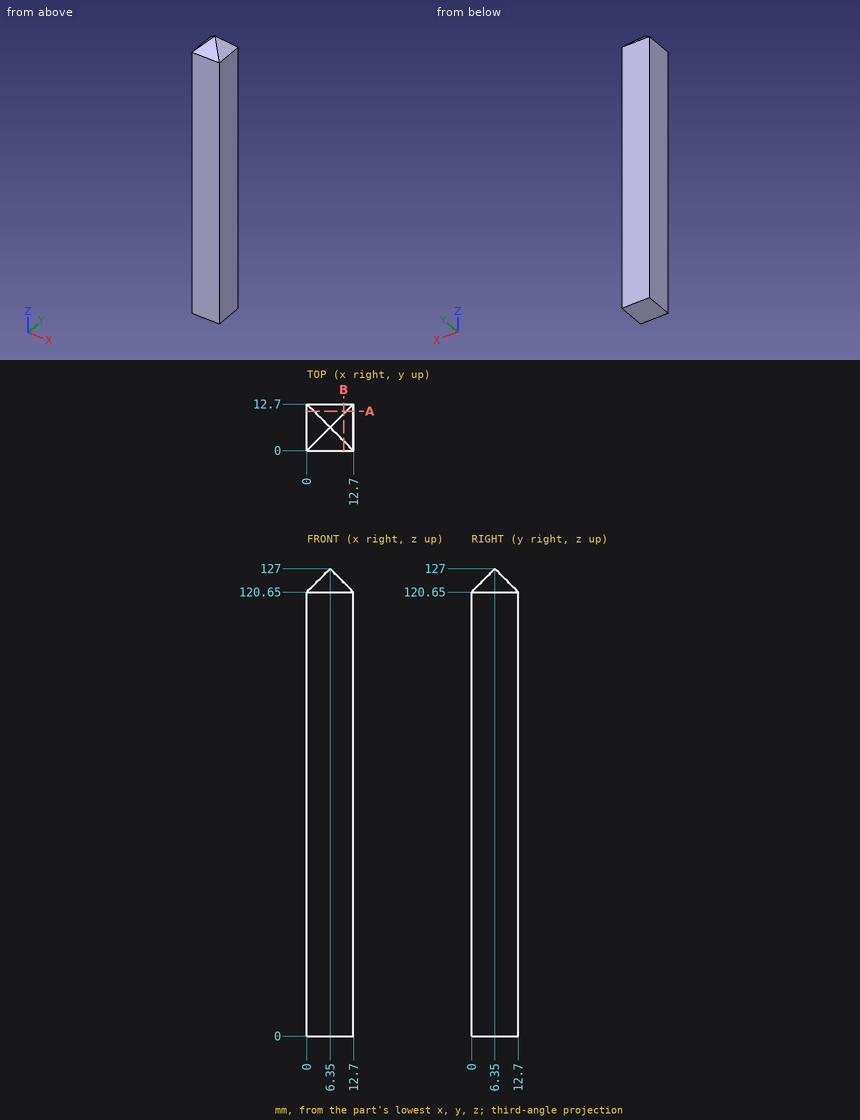
Geometry check sheet. Reference: drawing and pictorial views, mm from the part's lowest x, y, z. Give positions to 0.01 mm unless a question says otherwise; leave off trailing zeros. Loops run counter-clockwise (first coordinate to the right, second up) from the corner with the lowest first, then second, coordinate; pieces in that order, holes last.
1. Section check A-A, the plane y = 10.75. Enter the section's corners in (x, z), then the cut area to 3 significant figures.
2. Thickness scan on line 1 (Z direction, x = 7.25, y = 9.5); line 2 (Z direction, x = 1, y = 7); line 3 (Y direction, x = 9, z = 121). Record the ranges inside material, lowest first.
3. Section check B-B, the plane x = 10. Enter the section's corners in (y, z), then the cut area to 3 significant figures.
Geometry says:
1. outline: (0, 0) - (12.7, 0) - (12.7, 120.65) - (10.75, 122.6) - (1.95, 122.6) - (0, 120.65) - close
1. area: 1,550 mm2
2. line 1: z = 0 to 123.85
2. line 2: z = 0 to 121.65
2. line 3: y = 0.35 to 12.35
3. outline: (0, 0) - (12.7, 0) - (12.7, 120.65) - (10, 123.35) - (2.7, 123.35) - (0, 120.65) - close
3. area: 1,560 mm2
